CAD build for the part. Positions are in the model's coordinates, mm. Face numbers are marked on the shaded views. A direction names the side the tool comes from. Coordinates: 2 decimals unless noted, no trailing zeros. Loops run counter-clockwise (first coordinate to the right, second up) from the corner with the lowest first, then second, coordinate; pieces in that order, holes last. Notation, with made-up numbers: (73, 51) -> (102, 51) arc R18 ccw to (102, 62) -> close; hole circle Ø8 at (45, 64). An arc over 180 degrees is marked (long way). Return JSON: item names as keys, results as strings. Group by question number.
(1) Saw through at C-C on y = 12. Write the cut outline in (x, z), then the cut area to 3 significant figures.
(2) Saw through at A-A on z = 2.25. Write the cut outline in (x, y).
(3) Mould opens along X. For the marked faces 1, 2 and 3 say: pulls with the +X half, pulls with the -X half, needs draft (parallel to the pull), parting line crosses it, or undercut.
(4) Saw through at B-B on x = 1. Write the cut outline in (y, z), then the cut area to 3 significant figures.
(5) Tool access for the marked faces 4 and 5: list every direction of +Z, -Z, +X, -X, +Y, -Y with a clear straight run to the whole face (end or side of a thin tool).
(6) Probe L1, parallel to X at y = 80.5, z = -1.25; L2, parallel to Z at x = -11.5, y = 12. List the from-to ranges inside material, lowest first.
(7) Saw through at D-D on x = -10. Give the number of separate pieces and of enclosed holes in the cut face, then the cut area to 3 significant figures.
(8) Flat gauge pin, fed straight in: pin 1 Ø2.5 at (x, y) = (-10.32, 80.9) entering from +Z (3 decimals). Where does the tip first touch, or does it go through?
```python
from build123d import *

# Parameters (mm, degrees)
SKETCH_1_W          = 40
SKETCH_1_H          = 20
EXTRUDE_1_DEPTH     = 98
SHELL_1_T           = -1
SKETCH_2_R          = 1.5
CUT_EXTRUDE_1_DEPTH = 23
SKETCH_4_R          = 1.5
CUT_EXTRUDE_2_DEPTH = 48


with BuildPart() as part:
    # Sketch 1 → Extrude 1 (new body)
    with BuildSketch(Plane(origin=(0, 0, 0), x_dir=(1, 0, 0), z_dir=(0, 1, 0))):
        Rectangle(SKETCH_1_W, SKETCH_1_H)
    extrude(amount=EXTRUDE_1_DEPTH)

    # Shell 1
    shell_1_openings = [part.faces().sort_by_distance(p)[0] for p in [
        (0, 98, 0),
        (0, 0, 0),
    ]]
    offset(amount=SHELL_1_T, openings=shell_1_openings, kind=Kind.INTERSECTION)

    # Sketch 2 → Cut-Extrude 1 (cut)
    with BuildSketch(Plane(origin=(0, 0, -10), x_dir=(-1, 0, 0), z_dir=(0, 0, -1))):
        with Locations((-10.180049386, 8.687582917)):
            Circle(SKETCH_2_R)
        with Locations((-10.180049386, 21.401128756)):
            Circle(SKETCH_2_R)
        with Locations((10.180049386, 21.401128756)):
            Circle(SKETCH_2_R)
        with Locations((10.180049386, 8.687582917)):
            Circle(SKETCH_2_R)
    extrude(amount=-CUT_EXTRUDE_1_DEPTH, mode=Mode.SUBTRACT)

    # Sketch 4 → Cut-Extrude 2 (cut)
    with BuildSketch(Plane(origin=(0, 0, -10), x_dir=(-1, 0, 0), z_dir=(0, 0, -1))):
        with Locations((10.321220159, 60.899833626)):
            Circle(SKETCH_4_R)
        with Locations((-10.116242576, 60.899833626)):
            Circle(SKETCH_4_R)
        with Locations((-10.116242576, 70.899833626)):
            Circle(SKETCH_4_R)
        with Locations((10.321220159, 70.899833626)):
            Circle(SKETCH_4_R)
        with Locations((10.321220159, 80.899833626)):
            Circle(SKETCH_4_R)
        with Locations((-10.116242576, 80.899833626)):
            Circle(SKETCH_4_R)
        with Locations((10.321220159, 90.899833626)):
            Circle(SKETCH_4_R)
        with Locations((-10.116242576, 90.899833626)):
            Circle(SKETCH_4_R)
    extrude(amount=-CUT_EXTRUDE_2_DEPTH, mode=Mode.SUBTRACT)


solid = part.part
```
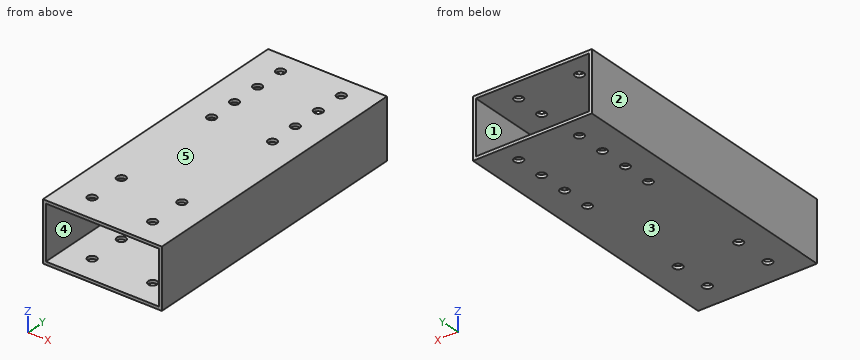
Geometry results:
{
 "1": {"outline": "(-20, -10) -> (20, -10) -> (20, 10) -> (-20, 10) -> close; hole (-19, -9) -> (19, -9) -> (19, 9) -> (-19, 9) -> close", "area": "116 mm²"},
 "2": {"outline": "(-20, 0) -> (-19, 0) -> (-19, 98) -> (-20, 98) -> close; (19, 0) -> (20, 0) -> (20, 98) -> (19, 98) -> close"},
 "3": {"face 1": "undercut", "face 2": "pulls with the -X half", "face 3": "needs draft"},
 "4": {"outline": "(0, -10) -> (98, -10) -> (98, -9) -> (0, -9) -> close; (0, 9) -> (98, 9) -> (98, 10) -> (0, 10) -> close", "area": "196 mm²"},
 "5": {"face 4": "+Y, -Y", "face 5": "+Z, +X, -X, +Y, -Y"},
 "6": {"L1": "-20 to -19, 19 to 20", "L2": "-10 to -9, 9 to 10"},
 "7": {"separate pieces": "14", "enclosed holes": "0", "area": "161 mm²"},
 "8": {"pin 1": "through"}
}
